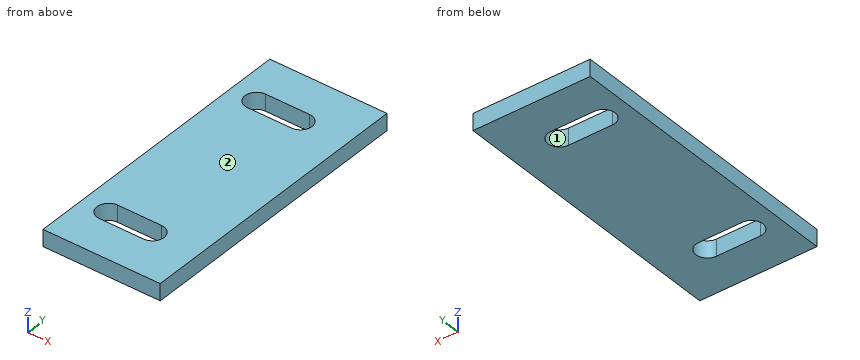
```python
from build123d import *

# Parameters (mm, degrees)
SKETCH1_W           = 28
SKETCH1_H           = 69
BOSS_EXTRUDE1_DEPTH = 4


with BuildPart() as part:
    # Sketch1 → Boss-Extrude1 (new body)
    with BuildSketch(Plane.XY.offset(4)):
        with Locations((-14, 0)):
            Rectangle(SKETCH1_W, SKETCH1_H)
        with BuildLine():
            Line((-21.75, 25.25), (-11.25, 25.25))
            ThreePointArc((-11.25, 25.25), (-8.5, 22.5), (-11.25, 19.75))
            Line((-11.25, 19.75), (-21.75, 19.75))
            ThreePointArc((-21.75, 19.75), (-24.5, 22.5), (-21.75, 25.25))
        make_face(mode=Mode.SUBTRACT)
        with BuildLine():
            Line((-21.75, -19.75), (-11.25, -19.75))
            ThreePointArc((-11.25, -19.75), (-8.5, -22.5), (-11.25, -25.25))
            Line((-11.25, -25.25), (-21.75, -25.25))
            ThreePointArc((-21.75, -25.25), (-24.5, -22.5), (-21.75, -19.75))
        make_face(mode=Mode.SUBTRACT)
    extrude(amount=-BOSS_EXTRUDE1_DEPTH)


solid = part.part
```
Geometry: final body of the model. Coordinates: model frame, mm. Face numbers are marked on the shaded views. A direction names the side the tool comes from. Round coordinates to 2 decimals unless told otherwise and drop trailing zeros. Loops run counter-clockwise (first coordinate to the right, second up) from the corner with the lowest first, then second, coordinate; pieces in that order, holes last. Notation, with made-up numbers: (-33.75, 77) -> (-13.75, 77) arc R25 cw to (-13.75, 114) -> close; hole circle Ø6 at (-24, -8). An arc over 180 degrees is marked (long way). Use one line per item in the form item = value. Start each with the question number.
1) Section B-B on x = -17.25. Output: boundary loops of the cut face in (y, z), then the cut area to 3 significant figures.
2) First-contact query: P1, Ø3, axis at x = -20.5, y = 16.5, coming from the -Z side. Flat tip, straight axial feed; report the tip coordinate or a pass-through.
3) Line query: L1, parallel to Y at x = -13.5, z = 3.15; L2, parallel to X at y = 22.5, z = 3.4; L3, parallel to Y at x = -10.25, z = 3.4. Output: solid intervals per line, ascending.
4) Section C-C on z = 2.15. Output: boundary loops of the cut face in (x, y), then the cut area to 3 significant figures.
5) Section A-A on y = -22.5. Output: boundary loops of the cut face in (x, z), then the cut area to 3 significant figures.
6) Access query for the marked faces 1 and 2. Directions: +Z, -Z, +X, -X, +Y, -Y. A direction counts if a zero-diameter tool reaches every point of the face in a straight line with its end or side. Return the directions, or none.
Response:
q1.outline = (-34.5, 0) -> (-25.25, 0) -> (-25.25, 4) -> (-34.5, 4) -> close; (-19.75, 0) -> (19.75, 0) -> (19.75, 4) -> (-19.75, 4) -> close; (25.25, 0) -> (34.5, 0) -> (34.5, 4) -> (25.25, 4) -> close
q1.area = 232 mm^2
q2.P1 = 0
q3.L1 = -34.5 to -25.25, -19.75 to 19.75, 25.25 to 34.5
q3.L2 = -28 to -24.5, -8.5 to 0
q3.L3 = -34.5 to -25.06, -19.94 to 19.94, 25.06 to 34.5
q4.outline = (-28, -34.5) -> (0, -34.5) -> (0, 34.5) -> (-28, 34.5) -> close; hole (-21.75, -25.25) -> (-11.25, -25.25) arc R2.75 ccw to (-11.25, -19.75) -> (-21.75, -19.75) arc R2.75 ccw to start; hole (-21.75, 19.75) -> (-11.25, 19.75) arc R2.75 ccw to (-11.25, 25.25) -> (-21.75, 25.25) arc R2.75 ccw to start
q4.area = 1,770 mm^2
q5.outline = (-28, 0) -> (-24.5, 0) -> (-24.5, 4) -> (-28, 4) -> close; (-8.5, 0) -> (0, 0) -> (0, 4) -> (-8.5, 4) -> close
q5.area = 48.0 mm^2
q6.face_1 = +Z, -Z
q6.face_2 = +Z, +X, -X, +Y, -Y
